Verification items for the finished model (mm, model axes). Face numbers are marked on the shaded views. A direction names the side the tool comes from. Give positions to 0.01 mm unless a question says otherwise; leave off trailing zeros. Order: outer loops, then holes, each group sorted by start corner. A loop starts at its lowest first (then second) coordinate and runs counter-clockwise, first axis right, second up.
(1) Gauge pin test, flat ends, axial feed: pin 1 (9.5 mm diameter, centred on x = 27.5, z = -11.5, fed in from +Y); pin 2 (1 mm diameter, centred on y = 22, z = 0.5, fed in from +X); pin 3 (1 mm diameter, centred on x = 0.5, y = 29.5, fed in from -Z). Record the tip position at first contact, or that the pin passes through.
(2) Sectioned sample at B-B on z = -25. Record the cut outline in (x, y), plus the area to 3 significant figures.
(3) Sectioned sample at D-D on x = 11. Record the cut outline in (y, z), plus the area to 3 significant figures.
(4) Sectioned sample at C-C on y = 20.6. Record the cut outline in (x, z), plus the area to 3 significant figures.
(5) Scan lines: L1, parallel to Z at x = 16, y = 18; L2, parallel to Z at x = 40, y = -0.2; L3, parallel to Y at x = 27, z = -9. Record each from-to range of solid material in increasing order.
(6) Mould release check, pull along Z, two halves, no side actions. Record for the marked faces 1, 2, 3 and 4: pulls with the +Z half, pulls with the -Z half, needs draft (parallel to the pull), parting line crosses it, or undercut.
(7) Access from +Z, -Z, +X, -X, +Y, -Y to the whole of each face (thin tool, end or side, straight path). Record for the marked faces 5, 6 and 7.
(8) Sectioned sample at A-A on y = 7.23. Record the cut outline in (x, z).
```python
from build123d import *

# Parameters (mm, degrees)
SKETCH1_W                    = 43
SKETCH1_H                    = 32
BASE_FLANGE1_DEPTH           = 0.91
EDGE_FLANGE1_STRIP_W         = 5.164
EDGE_FLANGE1_STRIP_H         = 0.91
EDGE_FLANGE1_STRIP_CUT_DEPTH = 32
EDGE_FLANGE1_DEPTH           = 32
EDGE_FLANGE2_STRIP_W         = 5.164
EDGE_FLANGE2_STRIP_H         = 0.91
EDGE_FLANGE2_STRIP_CUT_DEPTH = 34.738
EDGE_FLANGE2_DEPTH           = 34.738
SKETCH9_R                    = 4
MOTOR_HOLES_DEPTH            = 0.91
M3_CLEARANCE_HOLE3_D         = 3.4
M3_CLEARANCE_HOLE3_DEPTH     = 12
M3_CLEARANCE_HOLE3_TIP       = 1.021463052
SKETCH31_W                   = 8
SKETCH31_H                   = 20.5
CUT_EXTRUDE3_DEPTH           = 10
FILLET2_R                    = 5
SKETCH34_R                   = 1.4
CUT_EXTRUDE4_DEPTH           = 10
SKETCH35_R                   = 1.4
CUT_EXTRUDE5_DEPTH           = 10


# Sheet-metal steps are written as plain solids
with BuildPart() as part:
    # Sketch1 → Base-Flange1 (new body)
    with BuildSketch(Plane(origin=(0, 0, 0), x_dir=(1, 0, 0), z_dir=(0, 1, 0))):
        with Locations((21.5, 16)):
            Rectangle(SKETCH1_W, SKETCH1_H)
    extrude(amount=-BASE_FLANGE1_DEPTH)

    # Edge-Flange1 strip (across the edge) → Edge-Flange1 strip cut (cut)
    with BuildSketch(Plane.XY.offset(-32)):
        with Locations((-0.91, -0.455)):
            Rectangle(EDGE_FLANGE1_STRIP_W, EDGE_FLANGE1_STRIP_H)
    extrude(amount=EDGE_FLANGE1_STRIP_CUT_DEPTH, mode=Mode.SUBTRACT)

    # Edge-Flange1 section (across the edge) → Edge-Flange1 (add)
    with BuildSketch(Plane.XY.offset(-32)):
        with BuildLine():
            Line((0, 0.762), (0, 35.5))
            Line((0, 35.5), (0.91, 35.5))
            Line((0.91, 35.5), (0.91, 0.762))
            ThreePointArc((0.91, 0.762), (1.133184633, 0.223184633), (1.672, 0))
            Line((1.672, 0), (1.672, -0.91))
            ThreePointArc((1.672, -0.91), (0.489717462, -0.420282538), (0, 0.762))
        make_face()
    extrude(amount=EDGE_FLANGE1_DEPTH)

    # Edge-Flange2 strip (across the edge) → Edge-Flange2 strip cut (cut)
    with BuildSketch(Plane(origin=(0.91, 35.5, 0), x_dir=(0, 0, -1), z_dir=(0, -1, 0))):
        with Locations((-1.82, -0.455)):
            Rectangle(EDGE_FLANGE2_STRIP_W, EDGE_FLANGE2_STRIP_H)
    edge_flange2_strip_cut = extrude(amount=EDGE_FLANGE2_STRIP_CUT_DEPTH, mode=Mode.SUBTRACT)

    # Edge-Flange2 section (across the edge) → Edge-Flange2 (add)
    with BuildSketch(Plane(origin=(0.91, 35.5, 0), x_dir=(0, 0, -1), z_dir=(0, -1, 0))):
        with BuildLine():
            Line((-0.91, 0.762), (-0.91, 17))
            Line((-0.91, 17), (0, 17))
            Line((0, 17), (0, 0.762))
            ThreePointArc((0, 0.762), (0.223184633, 0.223184633), (0.762, 0))
            Line((0.762, 0), (0.762, -0.91))
            ThreePointArc((0.762, -0.91), (-0.420282538, -0.420282538), (-0.91, 0.762))
        make_face()
    edge_flange2 = extrude(amount=EDGE_FLANGE2_DEPTH)

    # Sketch9 → Motor Holes (cut)
    with BuildSketch(Plane.ZY):
        with Locations(Location((-12.5, 15, 0), (0, 0, 270))):
            Circle(SKETCH9_R)
    extrude(amount=-MOTOR_HOLES_DEPTH, mode=Mode.SUBTRACT)

    # Mirror4: Edge-Flange2 strip cut, Edge-Flange2 across plane
    add(edge_flange2_strip_cut.mirror(Plane(origin=(0, 0, -16), x_dir=(1, 0, 0), z_dir=(0, 0, -1))), mode=Mode.SUBTRACT)
    add(edge_flange2.mirror(Plane(origin=(0, 0, -16), x_dir=(1, 0, 0), z_dir=(0, 0, -1))))

    # M3 Clearance Hole3
    with Locations(Plane(origin=(0, 0, 0), x_dir=(1, 0, 0), z_dir=(0, 1, 0))):
        with Locations((40, 7), (4.672, 3), (40, 25)):
            Hole(M3_CLEARANCE_HOLE3_D / 2, depth=M3_CLEARANCE_HOLE3_DEPTH)
            with Locations((0, 0, -(M3_CLEARANCE_HOLE3_DEPTH + M3_CLEARANCE_HOLE3_TIP / 2))):  # 118° drill point
                Cone(0, M3_CLEARANCE_HOLE3_D / 2, M3_CLEARANCE_HOLE3_TIP, mode=Mode.SUBTRACT)

    # Sketch31 → Cut-Extrude3 (cut)
    with BuildSketch(Plane.ZY):
        with Locations((-12.5, 25.25)):
            Rectangle(SKETCH31_W, SKETCH31_H)
    extrude(amount=-CUT_EXTRUDE3_DEPTH, mode=Mode.SUBTRACT)

    # Fillet2
    fillet2_edges = [part.edges().sort_by_distance(p)[0] for p in [
        (43, -0.455, -32),
        (43, -0.455, 0),
    ]]
    fillet(fillet2_edges, radius=FILLET2_R)

    # Sketch34 → Cut-Extrude4 (cut)
    with BuildSketch(Plane.ZY):
        with Locations(Location((-7.1, 7.23, 0), (0, 0, 270))):
            Circle(SKETCH34_R)
    extrude(amount=-CUT_EXTRUDE4_DEPTH, mode=Mode.SUBTRACT)

    # Sketch35 → Cut-Extrude5 (cut)
    with BuildSketch(Plane.ZY):
        with Locations(Location((-21.08, 20.6, 0), (0, 0, 270))):
            Circle(SKETCH35_R)
    extrude(amount=-CUT_EXTRUDE5_DEPTH, mode=Mode.SUBTRACT)


solid = part.part
```
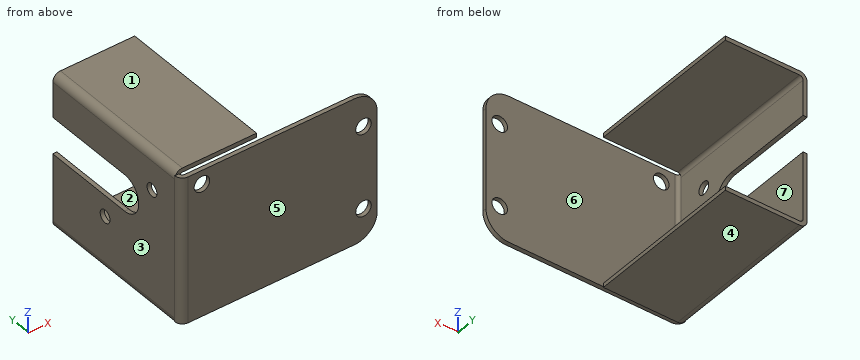
Ans:
1. pin 1: stops at y = 0
1. pin 2: stops at x = 17.91
1. pin 3: stops at z = -32.77
2. outline: (0, 0.76) arc R1.67 ccw to (1.67, -0.91) - (38.3, -0.91) - (38.3, 0) - (1.67, 0) arc R0.76 cw to (0.91, 0.76) - (0.91, 35.5) - (0, 35.5) - close; (41.7, -0.91) - (43, -0.91) - (43, 0) - (41.7, 0) - close
2. area: 67.9 mm2
3. outline: (-0.91, -32) - (0, -32) - (0, 0) - (-0.91, 0) - close; (0.76, -32.91) - (35.5, -32.91) - (35.5, -32) - (0.76, -32) - close; (0.76, 0) - (35.5, 0) - (35.5, 0.91) - (0.76, 0.91) - close
3. area: 92.3 mm2
4. outline: (0, -31.24) arc R1.67 ccw to (1.67, -32.91) - (17.91, -32.91) - (17.91, -32) - (1.67, -32) arc R0.76 cw to (0.91, -31.24) - (0.91, -22.48) - (0, -22.48) - close; (0, -19.68) - (0.91, -19.68) - (0.91, -16.5) - (0, -16.5) - close; (0, -8.5) - (0.91, -8.5) - (0.91, -0.76) arc R0.76 cw to (1.67, 0) - (17.91, 0) - (17.91, 0.91) - (1.67, 0.91) arc R1.67 ccw to (0, -0.76) - close
4. area: 50.9 mm2
5. L1: z = -32.91 to -32, 0 to 0.91
5. L2: z = -31.58 to -26.7, -23.3 to -8.7, -5.3 to -0.42
5. L3: y = -0.91 to 0
6. face 1: pulls with the +Z half
6. face 2: undercut
6. face 3: needs draft
6. face 4: pulls with the -Z half
7. face 5: +Z, -Z, +X, -X, -Y
7. face 6: +Z, -Z, +X, +Y
7. face 7: +X, +Y
8. outline: (0, -31.24) arc R1.67 ccw to (1.67, -32.91) - (17.91, -32.91) - (17.91, -32) - (1.67, -32) arc R0.76 cw to (0.91, -31.24) - (0.91, -8.5) - (0, -8.5) - close; (0, -5.7) - (0.91, -5.7) - (0.91, -0.76) arc R0.76 cw to (1.67, 0) - (17.91, 0) - (17.91, 0.91) - (1.67, 0.91) arc R1.67 ccw to (0, -0.76) - close
